```python
from build123d import *

# Parameters (mm, degrees)
F1_DEPTH      = 3
F2_R          = 15.7802685444
F3_DEPTH      = 15
F3_DEPTH_BACK = 5
F5_DEPTH      = 25
F7_DEPTH      = 1.5
F9_DEPTH      = 7
F10_R         = 1
F11_R         = 0.25
F12_DEPTH     = 60


with BuildPart() as f1:
    # F0 (on Top) → F1 (new body)
    with BuildSketch(Plane.XY):
        with BuildLine():
            Line((-10, -25), (10, -25))
            ThreePointArc((10, -25), (13.5355339059, -23.5355339059), (15, -20))
            Line((15, -20), (15, 20))
            ThreePointArc((15, 20), (13.5355339059, 23.5355339059), (10, 25))
            Line((10, 25), (-10, 25))
            ThreePointArc((-10, 25), (-13.5355339059, 23.5355339059), (-15, 20))
            Line((-15, 20), (-15, -20))
            ThreePointArc((-15, -20), (-13.5355339059, -23.5355339059), (-10, -25))
        make_face()
    extrude(amount=F1_DEPTH)

    # F2 (on Front) → F3 (cut, two sides)
    with BuildSketch(Plane.XZ) as f3_sk:
        with Locations((0, 13.2022947073)):
            Circle(F2_R)
    extrude(amount=-F3_DEPTH, mode=Mode.SUBTRACT)
    extrude(f3_sk.sketch, amount=F3_DEPTH_BACK, mode=Mode.SUBTRACT)

    # F4 (on face) → F5 (cut)
    with BuildSketch(Plane.XY.offset(3)):
        with BuildLine():
            ThreePointArc((11.1025739461, -15.6803686619), (10.5167875085, -14.2661550995), (9.1025739461, -13.6803686619))
            Line((9.1025739461, -13.6803686619), (-9.1025739461, -13.6803686619))
            ThreePointArc((-9.1025739461, -13.6803686619), (-10.5167875085, -14.2661550995), (-11.1025739461, -15.6803686619))
            Line((-11.1025739461, -15.6803686619), (-11.1025739461, -21.1788791716))
            ThreePointArc((-11.1025739461, -21.1788791716), (-10.5167875085, -22.593092734), (-9.1025739461, -23.1788791716))
            Line((-9.1025739461, -23.1788791716), (9.1025739461, -23.1788791716))
            ThreePointArc((9.1025739461, -23.1788791716), (10.5167875085, -22.593092734), (11.1025739461, -21.1788791716))
            Line((11.1025739461, -21.1788791716), (11.1025739461, -15.6803686619))
        make_face()
        with BuildLine():
            ThreePointArc((11.1025739461, 20.9576397687), (10.5167875085, 22.3718533311), (9.1025739461, 22.9576397687))
            Line((9.1025739461, 22.9576397687), (-9.1025739461, 22.9576397687))
            ThreePointArc((-9.1025739461, 22.9576397687), (-10.5167875085, 22.3718533311), (-11.1025739461, 20.9576397687))
            Line((-11.1025739461, 20.9576397687), (-11.1025739461, 18.9862303883))
            ThreePointArc((-11.1025739461, 18.9862303883), (-10.5167875085, 17.5720168259), (-9.1025739461, 16.9862303883))
            Line((-9.1025739461, 16.9862303883), (9.1025739461, 16.9862303883))
            ThreePointArc((9.1025739461, 16.9862303883), (10.5167875085, 17.5720168259), (11.1025739461, 18.9862303883))
            Line((11.1025739461, 18.9862303883), (11.1025739461, 20.9576397687))
        make_face()
    extrude(amount=-F5_DEPTH, mode=Mode.SUBTRACT)

    # F6 (on face) → F7 (cut)
    with BuildSketch(Plane(origin=(0, 0, 0), x_dir=(1, 0, 0), z_dir=(0, 0, -1))):
        Polygon((8.6438585016, 5), (3.1369663253, 13.6803686619), (-2.8630336747, 13.6803686619), (-8.6438585016, 5), align=None)
        Polygon((-6.5296259269, -16.9862303883), (-4.6438585016, -15), (-8.6438585016, -15), (-6.8296259269, -16.9862303883), align=None)
        Polygon((-0.2438585016, -15), (-4.2438585016, -15), (-2.4296259269, -16.9862303883), (-2.1296259269, -16.9862303883), align=None)
        Polygon((4.1561414984, -15), (0.1561414984, -15), (1.9703740731, -16.9862303883), (2.2703740731, -16.9862303883), align=None)
        Polygon((8.5561414984, -15), (4.5561414984, -15), (6.3703740731, -16.9862303883), (6.6703740731, -16.9862303883), align=None)
    extrude(amount=-F7_DEPTH, mode=Mode.SUBTRACT)

    # F8 (on face) → F9 (join)
    with BuildSketch(Plane(origin=(-15, 0, 0), x_dir=(0, -1, 0), z_dir=(-1, 0, 0))):
        Polygon((-13.7345343828, 3), (-16.5546499193, 3), (-16.3944102824, 1.7589493655), (-13.7345343828, 2.1682542283), align=None)
        Polygon((-10.7979638994, 3), (-13.4345343828, 3), (-13.4345343828, 2.1682542283), (-10.7979638994, 1.8060837174), align=None)
    extrude(amount=-F9_DEPTH)

    # F10
    f10_edges = [f1.edges().sort_by_distance(p)[0] for p in [
        (-8, 10.797964, 2.403042),
        (-8, 13.434534, 2.584127),
        (-8, 13.734534, 2.584127),
    ]]
    fillet(f10_edges, radius=F10_R)

    # F11 (on face) → F12 (cut)
    with BuildSketch(Plane.XZ.offset(25)):
        with Locations((0, 1.1609706562)):
            Circle(F11_R)
    extrude(amount=-F12_DEPTH, mode=Mode.SUBTRACT)


solid = f1.part
```
The listing builds one solid part. Answer for the finished solid, in the listing's coordinates (mm). A direction names the side the tool comes from. Give positions to 0.01 mm unless a question says otherwise; leave off trailing zeros. Order: outer loops, then holes, each group sorted by start corner. A loop starts at its lowest first (then second) coordinate and runs counter-clockwise, first axis right, second up. Notation, with made-up numbers: (80.5, 68.25) - (138.5, 68.25) arc R20 cw to (138.5, 91.25) - close; hole circle Ø6 at (-3.75, 36.25). An arc over 180 degrees is marked (long way). Answer in a Markdown table with one row per item. Add a question column.
Q1. The part is cut by section A-A (y = 7). Determine the outline of the cut face in (x, z), then the cut area to 3 significant figures.
Q2. For a pull along X with two mould halves and no side action, classify faces 1 (the flat face through (0, -5, 2)), 2 (the cylindrical face through (-13, 24, 1)), 3 (the flat face through (0, -25, 2)) as released by +X, released by -X, zero draft, split by the parting line, or undercut.
Q3. Which of the six approach directions +Z, -Z, +X, -X, +Y, -Y give full straight-line access (tool end or side, diameter ignored) to faces 4 (the cylindrical face through (10.43, 5.14, 1.36)), 5 (the flat face through (0, 16.986, 2)), 6 (the flat face through (-9.66, 12.13, 1.99))?
Q4. The part is cut by section B-B (x = -5.25). Determine the outline of the cut face in (y, z).
Q5. Given P1, Ø0.9, axis at x = -11, z = 2.5, coming from the +Y side; P2, Ø4.5, axis at x = 1, y = -8, coming from the -Z side, each flat-ended and moving along its own axis, determine where each tip first touches the part or whether it passes through.
Q6. Find the intervals of material crossed by line 1 along Y through (x, z) = (1.25, 2.25); line 2 along Z through (x, y) = (0, 15.85); line 3 along X through (y, z) = (19, 0.5), in increasing order. Write a range as [from, to].
Determined:
| question | item | result |
|---|---|---|
| 1 | outline | (-15, 0) - (-8.64, 0) arc R15.78 cw to (-12.04, 3) - (-15, 3) - close; (8.64, 0) - (15, 0) - (15, 3) - (12.04, 3) arc R15.78 cw to start |
| 1 | area | 27.0 mm² |
| 2 | face 1 | undercut |
| 2 | face 2 | released by -X |
| 2 | face 3 | zero draft |
| 3 | face 4 | +Z |
| 3 | face 5 | +Z, -Z |
| 3 | face 6 | none |
| 4 | outline | (-25, 0) - (-23.18, 0) - (-23.18, 3) - (-25, 3) - close; (-13.68, 0) - (-10.1, 0) - (-10.1, 1.5) - (-5, 1.5) - (-5, 3) - (-13.68, 3) - close; (15, 1.5) - (15.64, 1.5) - (15.64, 0) - (16.99, 0) - (16.99, 3) - (15, 3) - close; (22.96, 0) - (25, 0) - (25, 3) - (22.96, 3) - close |
| 5 | P1 | stops at y = 24.97 |
| 5 | P2 | stops at z = 1.5 |
| 6 | line 1 | y = [-25, -23.18], [-13.68, -5], [15, 16.99], [22.96, 25] |
| 6 | line 2 | z = [0, 0.91], [1.41, 3] |
| 6 | line 3 | x = [-15, -11.1], [11.1, 15] |
